```python
from build123d import *

# Parameters (mm, degrees)
EXTRUDE_1_DEPTH     = 130
EXTRUDE_1_2_DEPTH   = 130
SKETCH_3_W          = 1
SKETCH_3_H          = 5
CUT_EXTRUDE_3_DEPTH = 166.227116419
SKETCH_5_W          = 200
SKETCH_5_H          = 15
EXTRUDE_2_DEPTH     = 170
SKETCH_6_W          = 15
SKETCH_6_H          = 115
EXTRUDE_3_DEPTH     = 150
CUT_EXTRUDE_4_DEPTH = 280.55321497
SKETCH_8_W          = 80
SKETCH_8_H          = 60
SKETCH_8_R          = 15
EXTRUDE_4_DEPTH     = 30
FILLET_1_R          = 30
FILLET_3_R          = 20
SKETCH_9_W          = 200
SKETCH_9_H          = 15
EXTRUDE_5_DEPTH     = 5
SKETCH_10_W         = 200
SKETCH_10_H         = 5
CUT_EXTRUDE_5_DEPTH = 2
SKETCH_11_W         = 200
SKETCH_11_H         = 10
CUT_EXTRUDE_6_DEPTH = 3


with BuildPart() as part:
    # Sketch 1 → Extrude 1 (new body)
    with BuildSketch(Plane(origin=(0, 0, 0), x_dir=(1, 0, 0), z_dir=(0, 1, 0))):
        Polygon((-60, 0), (-60, 20), (-65, 20), (-65, 0), (-73, 0), (-73, 5), (-70, 5), (-70, 10), (-90, 10), (-90, 5), (-87, 5), (-87, 0), (-95, 0), (-95, 20), (-100, 20), (-100, -5), (-60, -5), align=None)
    extrude(amount=EXTRUDE_1_DEPTH)


with BuildPart() as body_2:
    # Sketch 1 → Extrude 1 2 (new body)
    with BuildSketch(Plane(origin=(0, 0, 0), x_dir=(1, 0, 0), z_dir=(0, 1, 0))):
        Polygon((73, 0), (73, 5), (70, 5), (70, 10), (90, 10), (90, 5), (87, 5), (87, 0), (95, 0), (95, 20), (100, 20), (100, -5), (60, -5), (60, 0), (60, 20), (65, 20), (65, 0), align=None)
    extrude(amount=EXTRUDE_1_2_DEPTH)


with BuildPart() as cut_extrude_3_tool:
    # Sketch 3 → Cut-Extrude 3 (new, through all)
    with BuildSketch(Plane(origin=(0, 130, 0), x_dir=(1, 0, 0), z_dir=(0, 1, 0))):
        with Locations((-99.5, 12.5)):
            Rectangle(SKETCH_3_W, SKETCH_3_H)
        with Locations((-99.5, 2.5)):
            Rectangle(SKETCH_3_W, SKETCH_3_H)
        with Locations((-60.5, 12.5)):
            Rectangle(SKETCH_3_W, SKETCH_3_H)
        with Locations((-60.5, 2.5)):
            Rectangle(SKETCH_3_W, SKETCH_3_H)
        with Locations((60.5, 2.5)):
            Rectangle(SKETCH_3_W, SKETCH_3_H)
        with Locations((60.5, 12.5)):
            Rectangle(SKETCH_3_W, SKETCH_3_H)
        with Locations((99.5, 2.5)):
            Rectangle(SKETCH_3_W, SKETCH_3_H)
        with Locations((99.5, 12.5)):
            Rectangle(SKETCH_3_W, SKETCH_3_H)
    extrude(amount=-CUT_EXTRUDE_3_DEPTH)


with BuildPart() as part_1:
    add(part.part)

    # Cut-Extrude 3: cut by cut_extrude_3_tool
    add(cut_extrude_3_tool.part, mode=Mode.SUBTRACT)



with BuildPart() as body_2_1:
    add(body_2.part)

    # Cut-Extrude 3: cut by cut_extrude_3_tool
    add(cut_extrude_3_tool.part, mode=Mode.SUBTRACT)


with BuildPart() as part_2:
    add(part_1.part)

    add(body_2_1.part)  # Extrude 2 merges body 2
    # Sketch 5 → Extrude 2 (add)
    with BuildSketch(Plane.XY.offset(5)):
        with Locations((0, 122.5)):
            Rectangle(SKETCH_5_W, SKETCH_5_H)
    extrude(amount=EXTRUDE_2_DEPTH)

    # Sketch 6 → Extrude 3 (add)
    with BuildSketch(Plane.XY.offset(5)):
        with Locations((-67.5, 57.5)):
            Rectangle(SKETCH_6_W, SKETCH_6_H)
        with Locations((67.5, 57.5)):
            Rectangle(SKETCH_6_W, SKETCH_6_H)
    extrude(amount=EXTRUDE_3_DEPTH)

    # Sketch 7 → Cut-Extrude 4 (cut, through all)
    with BuildSketch(Plane.ZY.offset(75)):
        Polygon((25, 0), (155, 90), (155, 0), align=None)
    extrude(amount=-CUT_EXTRUDE_4_DEPTH, mode=Mode.SUBTRACT)

    # Sketch 8 → Extrude 4 (add)
    with BuildSketch(Plane(origin=(0, 130, 0), x_dir=(1, 0, 0), z_dir=(0, 1, 0))):
        with Locations((0, 25)):
            Rectangle(SKETCH_8_W, SKETCH_8_H)
        with Locations(Location((0, 20, 0), (0, 0, 270))):
            Circle(SKETCH_8_R, mode=Mode.SUBTRACT)
    extrude(amount=-EXTRUDE_4_DEPTH)

    # Fillet 1
    # the kernel refuses this fillet: 30 mm, written as the material it adds along each edge
    with BuildSketch(Plane(origin=(40, 130, 5), x_dir=(1, 0, 0), z_dir=(0, -1, 0))) as fillet_1_piece_1:
        with BuildLine():
            CenterArc((30, -28.284271247), FILLET_1_R, 109.471220634, 70.528779366)
            Line((0, -28.284271247), (0, 0))
            Line((0, 0), (20, 0))
        make_face()
    extrude(amount=15)
    with BuildSketch(Plane(origin=(-40, 130, 5), x_dir=(-1, 0, 0), z_dir=(0, -1, 0))) as fillet_1_piece_2:
        with BuildLine():
            CenterArc((30, 28.284271247), FILLET_1_R, 180, 70.528779366)
            Line((0, 28.284271247), (0, 0))
            Line((0, 0), (20, 0))
        make_face()
    extrude(amount=15)

    # Fillet 3
    fillet_3_edges = [part_2.edges().sort_by_distance(p)[0] for p in [
        (40, 107.5, 5),
        (-40, 107.5, 5),
        (-40, 115, -55),
        (40, 115, -55),
    ]]
    fillet(fillet_3_edges, radius=FILLET_3_R)

    # Sketch 9 → Extrude 5 (add)
    with BuildSketch(Plane(origin=(0, 130, 0), x_dir=(1, 0, 0), z_dir=(0, 1, 0))):
        with Locations((0, -147.5)):
            Rectangle(SKETCH_9_W, SKETCH_9_H)
        with Locations((0, -27.5)):
            Rectangle(SKETCH_9_W, SKETCH_9_H)
    extrude(amount=EXTRUDE_5_DEPTH)

    # Sketch 10 → Cut-Extrude 5 (cut)
    with BuildSketch(Plane(origin=(0, 135, 0), x_dir=(1, 0, 0), z_dir=(0, 1, 0))):
        with Locations((0, -27.241970949)):
            Rectangle(SKETCH_10_W, SKETCH_10_H)
        with Locations((0, -147.5)):
            Rectangle(SKETCH_10_W, SKETCH_10_H)
    extrude(amount=-CUT_EXTRUDE_5_DEPTH, mode=Mode.SUBTRACT)

    # Sketch 11 → Cut-Extrude 6 (cut)
    with BuildSketch(Plane(origin=(0, 133, 0), x_dir=(1, 0, 0), z_dir=(0, 1, 0))):
        with Locations((0, -27.370985475)):
            Rectangle(SKETCH_11_W, SKETCH_11_H)
        with Locations((0, -147.5)):
            Rectangle(SKETCH_11_W, SKETCH_11_H)
    extrude(amount=-CUT_EXTRUDE_6_DEPTH, mode=Mode.SUBTRACT)


solid = part_2.part
```
For this review, take the finished solid that the model builds, in its own axes (mm). A direction names the side the tool comes from. Round coordinates to 2 decimals unless told otherwise and drop trailing zeros. Write each loop counter-clockwise with the first axis right and the second up, starting at its lowest first coordinate (ties: lowest second). Pieces come first, ordered by that corner, then holes.
1) Machinability: for faces 5 (the face through (40, 112, -27)), 6 (the face through (-68, 103, 155)), 7 (the face through (80, 64, -10)), 8 (the face through (88, 57, 5)), which of the approach directions +Z, -Z, +X, -X, +Y, -Y give a long, thin tool a straight path to every point of the face, cutting with its end or side? Answer none if there is none.
Answer below:
face 5: -Z, -Y
face 6: +Z, +X, -X, -Y
face 7: -Z, +Y, -Y
face 8: +Z, +X, -Y
2) For line 1 along X through (y, z) = (97, 138.5); line 2 along X through (y, z) = (109, 1.5); line 3 along Y through (x, z) = (91.5, 33), list the stretches that pass through material, from the lowest coordinate up.
Answer below:
line 1: x = -75 to -60, 60 to 75
line 2: x = -100 to -60, -31.3 to 31.3, 60 to 100
line 3: y = 115 to 135
3) Take a section at A-A on z = 17. Give the boundary of the cut face in (x, y).
Answer below:
outline: (-100, 115) - (-75, 115) - (-75, 0) - (-60, 0) - (-60, 115) - (60, 115) - (60, 0) - (75, 0) - (75, 115) - (100, 115) - (100, 130) - (-100, 130) - close
4) Take a section at C-C on x = 48. Give the boundary of the cut face in (y, z).
Answer below:
outline: (115, -2.89) - (130, -2.89) - (130, 20) - (135, 20) - (135, 24.74) - (133, 24.74) - (133, 22.37) - (130, 22.37) - (130, 32.37) - (133, 32.37) - (133, 29.74) - (135, 29.74) - (135, 35) - (130, 35) - (130, 140) - (135, 140) - (135, 145) - (133, 145) - (133, 142.5) - (130, 142.5) - (130, 152.5) - (133, 152.5) - (133, 150) - (135, 150) - (135, 155) - (130, 155) - (130, 175) - (115, 175) - close
5) Insertion check: pin 1 Ø1.6 at (x, y) = (-3, 133.5) entering from +Z; pin 2 Ø16 at (y, z) = (64, -11) entering from -X; pin 3 Ø1.5 at (y, z) = (83.5, -13) entering from -X; pin 4 Ø1.2 at (x, z) = (36.5, 151.5) entering from -Y. Each pin has a flat end and moves straight along its axis. Give the tip position at first contact, or say it passes through.
Answer below:
pin 1: stops at z = 155
pin 2: stops at x = -100
pin 3: stops at x = -99
pin 4: stops at y = 115
6) Take a section at D-D on z = 90.5. Give the boundary of the cut face in (x, y).
Answer below:
outline: (-100, 115) - (-75, 115) - (-75, 45.35) - (-60, 45.35) - (-60, 115) - (60, 115) - (60, 45.35) - (75, 45.35) - (75, 115) - (100, 115) - (100, 130) - (-100, 130) - close
7) Mouldability with a two-part tool opening along X and no side actions: class faces 1 (the face through (75, 69, 62)), 2 (the face through (-45.357, 122.605, -6.175)), 3 (the face through (-60, 64, 59)), 4 (the face through (-1, 130, 27)) as +X half, -X half, draft (parallel to the pull), parting line (faces both ways), or undercut.
Answer below:
face 1: +X half
face 2: undercut
face 3: undercut
face 4: draft
